Geometry: final body of the model. Coordinates: model frame, mm. Face numbers are marked on the shaded views. A direction names the side the tool comes from. Coordinates: 2 decimals unless noted, no trailing zeros. Order: outer loops, then holes, each group sorted by start corner. A loop starts at its lowest first (then second) coordinate and runs counter-clockwise, first axis right, second up. Notation, with made-up numbers: (-35.5, 59) - (1.5, 59) arc R9 ccw to (1.5, 63) - close; hole circle Ø7 at (57.5, -24.75). An arc over 180 degrees is marked (long way). Use a Markdown table: item, result. Add a question column.
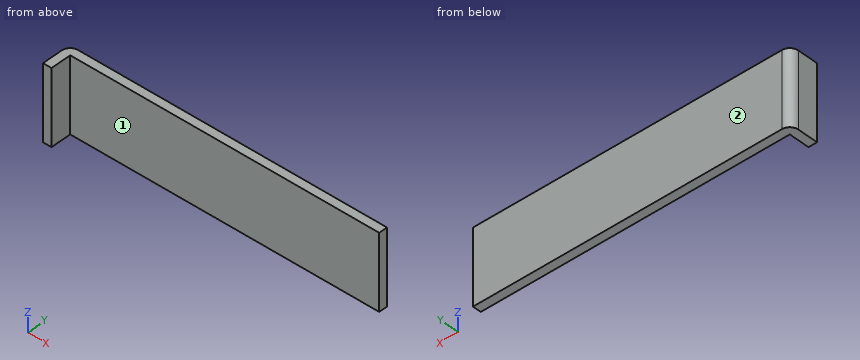
```python
from build123d import *

# Parameters (mm, degrees)
BOSS_EXTRU_1_DEPTH = 4.4
CONG_1_R           = 0.5


with BuildPart() as part:
    # Esquisse1 → Boss.-Extru.1 (new body)
    with BuildSketch(Plane.XY):
        Polygon((0, 0), (0, 1.7), (18.7, 1.7), (18.7, 1.2), (0.5, 1.2), (0.5, 0), align=None)
    extrude(amount=BOSS_EXTRU_1_DEPTH)

    # Congé1
    cong_1_edges = [part.edges().sort_by_distance(p)[0] for p in [
        (0, 1.7, 2.2),
    ]]
    fillet(cong_1_edges, radius=CONG_1_R)


solid = part.part
```
1) Line query: line 1 (X direction, y = 0.6, z = 0.45); line 2 (Y direction, x = 11, z = 2.2); line 3 (X direction, y = 1.6, z = 2.1). Output: solid intervals per line, ascending. Write a range as from..to.
2) Section query C-C (y = 0.95). Return the cut outline in (x, z).
3) Access query for the marked faces 1 and 2. Directions: +Z, -Z, +X, -X, +Y, -Y. A direction counts if a zero-diameter tool reaches every point of the face in a straight line with its end or side. Return the directions, or none.
4) Section query A-A (z = 1.65). Return the cut outline in (x, y).
5) Section query B-B (x = 3.25). Return the cut outline in (y, z).
From the geometry:
| question | item | result |
|---|---|---|
| 1 | line 1 | x = 0..0.5 |
| 1 | line 2 | y = 1.2..1.7 |
| 1 | line 3 | x = 0.2..18.7 |
| 2 | outline | (0, 0) - (0.5, 0) - (0.5, 4.4) - (0, 4.4) - close |
| 3 | face 1 | +Z, -Z, +X, -Y |
| 3 | face 2 | +Z, -Z, +X, -X, +Y |
| 4 | outline | (0, 0) - (0.5, 0) - (0.5, 1.2) - (18.7, 1.2) - (18.7, 1.7) - (0.5, 1.7) arc R0.5 ccw to (0, 1.2) - close |
| 5 | outline | (1.2, 0) - (1.7, 0) - (1.7, 4.4) - (1.2, 4.4) - close |
